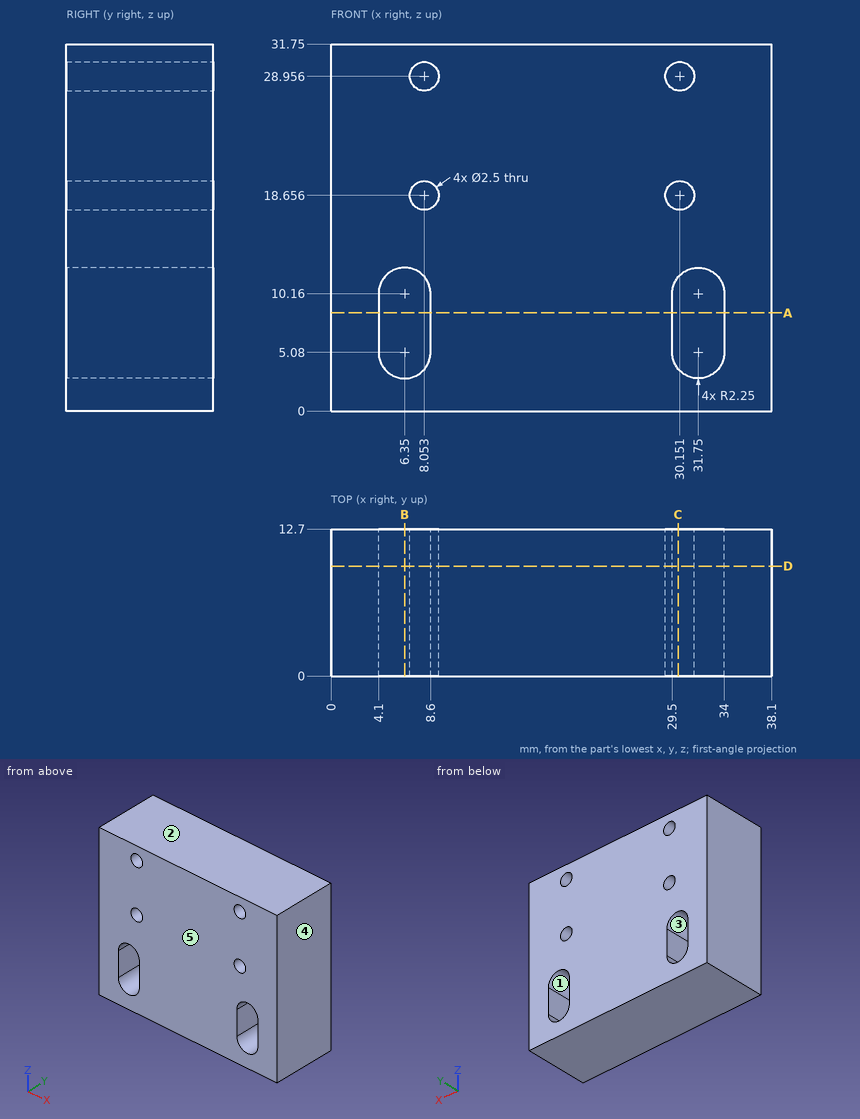
Study the drawing (mm; zero at the part's minimum x, y, z) and answer. A direction names the side the tool comes from. Round coordinates to 2 decimals unless told otherwise and drop trailing zeros. Loops run counter-clockwise (first coordinate to the right, second up) from the corner with the lowest first, then second, coordinate; pieces in that order, holes last. Notation, with made-up numbers: (-30, 13) -> (-7, 13) arc R21 cw to (-7, 41) -> close; hole circle Ø1 at (32, 62). An arc over 180 degrees is marked (long way). Use one line per item in the form item = value.
1. The part is cut by section B-B on x = 6.35. Determine the outline of the cut face in (y, z).
Answer key:
outline = (0, 0) -> (12.7, 0) -> (12.7, 2.83) -> (0, 2.83) -> close; (0, 12.41) -> (12.7, 12.41) -> (12.7, 31.75) -> (0, 31.75) -> close
2. For a pull along X with two mould halves and no side action, classify the marked faces 3, 4 and 5 as released by +X, released by -X, zero draft, split by the parting line, or undercut.
Answer key:
face_3 = undercut
face_4 = released by +X
face_5 = zero draft
3. The part is cut by section D-D on y = 9.5. Determine the outline of the cut face in (x, z).
Answer key:
outline = (0, 0) -> (38.1, 0) -> (38.1, 31.75) -> (0, 31.75) -> close; hole (4.1, 5.08) arc R2.25 ccw to (8.6, 5.08) -> (8.6, 10.16) arc R2.25 ccw to (4.1, 10.16) -> close; hole circle Ø2.5 at (8.05, 18.66); hole circle Ø2.5 at (8.05, 28.96); hole circle Ø2.5 at (30.15, 18.66); hole circle Ø2.5 at (30.15, 28.96); hole (29.5, 5.08) arc R2.25 ccw to (34, 5.08) -> (34, 10.16) arc R2.25 ccw to (29.5, 10.16) -> close
4. A tool of negligible diameter and unlimited length cuts with its end or side. For the marked faces 1 and 2, from which of +Z, -Z, +X, -X, +Y, -Y can it reach the whole face along a straight path? Write none if from no direction.
Answer key:
face_1 = +Y, -Y
face_2 = +Z, +X, -X, +Y, -Y
5. The part is cut by section A-A on z = 8.5. Determine the outline of the cut face in (x, y).
Answer key:
outline = (0, 0) -> (4.1, 0) -> (4.1, 12.7) -> (0, 12.7) -> close; (8.6, 0) -> (29.5, 0) -> (29.5, 12.7) -> (8.6, 12.7) -> close; (34, 0) -> (38.1, 0) -> (38.1, 12.7) -> (34, 12.7) -> close
6. The part is cut by section C-C on x = 30. Give the number of separate pieces and of enclosed holes in the cut face, and give its area (3 significant figures).
Answer key:
separate_pieces = 4
enclosed_holes = 0
area = 240 mm²
7. A flat-ended cylindrical pin translates along its axis: pin 1 Ø2 at (x, z) = (8.05, 28.96) entering from -Y. Find the tip coordinate at first contact, or state that the pin passes through.
Answer key:
pin_1 = through
8. Find the intervals of material crossed by probe 1 along X at (y, z) = (11.5, 18.5); probe 2 along X at (y, z) = (6.75, 6.5); probe 3 along Z at (x, y) = (5.5, 10.75), in increasing order. Write a range as [from, to].
Answer key:
probe_1 = [0, 6.81], [9.29, 28.91], [31.39, 38.1]
probe_2 = [0, 4.1], [8.6, 29.5], [34, 38.1]
probe_3 = [0, 3], [12.24, 31.75]
